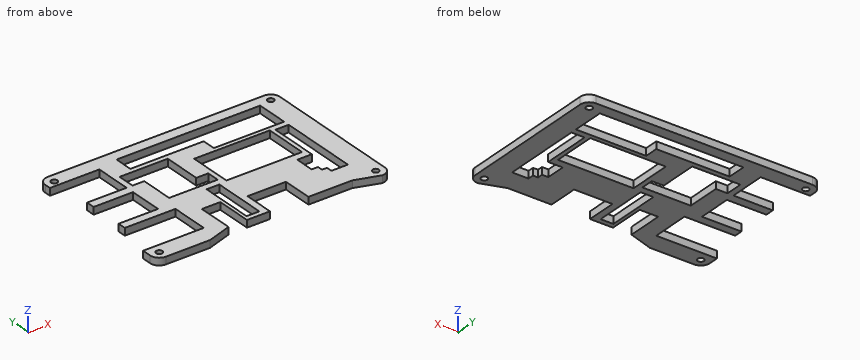
```python
from build123d import *

# Parameters (mm, degrees)
SKETCH2_W           = 5.4034
SKETCH2_H           = 22.6066
SKETCH2_W_2         = 31.9679
SKETCH2_H_2         = 18.2371
BOSS_EXTRUDE1_DEPTH = 3.048
SKETCH3_R           = 1.338245378
CUT_EXTRUDE1_DEPTH  = 72.310891511


with BuildPart() as part:
    # Sketch2 → Boss-Extrude1 (new body)
    with BuildSketch(Plane(origin=(0, 0, 8.171752382), x_dir=(-1, 0, 0), z_dir=(0, 0, -1))):
        with BuildLine():
            Line((-23.844892625, -33.084405696), (-34.084892625, -36.451005696))
            ThreePointArc((-34.084892625, -36.451005696), (-36.778969461, -35.335082532), (-37.894892625, -32.641005696))
            Line((-37.894892625, -32.641005696), (-37.894892625, 26.697694304))
            ThreePointArc((-37.894892625, 26.697694304), (-36.778969461, 29.391771141), (-34.084892625, 30.507694304))
            Line((-34.084892625, 30.507694304), (57.404932375, 30.507694304))
            ThreePointArc((57.404932375, 30.507694304), (60.103884597, 29.386886916), (61.214907375, 26.683892153))
            Line((61.214907375, 26.683892153), (61.214907375, 24.068294304))
            Line((61.214907375, 24.068294304), (40.325007375, 24.068294304))
            Line((40.325007375, 24.068294304), (40.325007375, 8.658194304))
            Line((40.325007375, 8.658194304), (56.975007375, 8.658194304))
            Line((56.975007375, 8.658194304), (56.975007375, 4.997894304))
            Line((56.975007375, 4.997894304), (40.325007375, 4.997894304))
            Line((40.325007375, 4.997894304), (40.325007375, -9.121805696))
            Line((40.325007375, -9.121805696), (56.975007375, -9.121805696))
            Line((56.975007375, -9.121805696), (56.975007375, -12.628005696))
            Line((56.975007375, -12.628005696), (35.575007375, -12.628005696))
            Line((35.575007375, -12.628005696), (35.575007375, -28.627805696))
            Line((35.575007375, -28.627805696), (61.214907375, -28.627805696))
            Line((61.214907375, -28.627805696), (61.214907375, -32.613401529))
            ThreePointArc((61.214907375, -32.613401529), (60.108826144, -35.325305244), (57.405007375, -36.451005696))
            Line((57.405007375, -36.451005696), (38.714307375, -36.451005696))
            Line((38.714307375, -36.451005696), (28.474307375, -33.084405696))
            Line((28.474307375, -33.084405696), (28.474307375, -18.034905696))
            Line((28.474307375, -18.034905696), (20.658107375, -18.034905696))
            Line((20.658107375, -18.034905696), (20.658107375, -33.084405696))
            Line((20.658107375, -33.084405696), (10.926407375, -33.084405696))
            Line((10.926407375, -33.084405696), (10.926407375, -20.384405696))
            Line((10.926407375, -20.384405696), (-5.302892625, -20.384405696))
            Line((-5.302892625, -20.384405696), (-5.302892625, -33.084405696))
            Line((-5.302892625, -33.084405696), (-23.844892625, -33.084405696))
        make_face()
        with Locations((16.546707375, -19.663505696)):
            Rectangle(SKETCH2_W, SKETCH2_H, mode=Mode.SUBTRACT)
        Polygon((-29.004892625, -23.698905696), (-22.066892625, -23.698905696), (-22.066892625, -21.185805696), (-19.950892625, -21.185805696), (-19.950892625, -18.920605696), (-17.244692625, -18.920605696), (-17.244692625, -10.792605696), (-23.416892625, -10.792605696), (-23.416892625, 9.801194304), (-29.004892625, 9.801194304), align=None, mode=Mode.SUBTRACT)
        with Locations((-5.654942625, 1.475544304)):
            Rectangle(SKETCH2_W_2, SKETCH2_H_2, mode=Mode.SUBTRACT)
        Polygon((12.361007375, -0.097605696), (17.441007375, -0.097605696), (17.441007375, 15.972394304), (37.825007375, 15.972394304), (37.825007375, 8.658194304), (32.872007375, 8.658194304), (32.872007375, -5.431505696), (12.361007375, -5.431505696), align=None, mode=Mode.SUBTRACT)
        Polygon((0.677107375, 12.372094304), (-29.004794688, 12.372094304), (-29.004892625, 25.896994304), (31.688307375, 25.896994304), (31.688307375, 18.086994304), (0.677107375, 18.086994304), align=None, mode=Mode.SUBTRACT)
    extrude(amount=BOSS_EXTRUDE1_DEPTH)

    # Sketch3 → Cut-Extrude1 (cut, through all)
    with BuildSketch(Plane(origin=(0, 0, 5.123752382), x_dir=(-1, 0, 0), z_dir=(0, 0, -1))):
        with Locations((57.405007375, -32.641005696)):
            Circle(SKETCH3_R)
        with Locations((-34.084892625, -32.641005696)):
            Circle(SKETCH3_R)
        with Locations((-34.084892625, 26.697694304)):
            Circle(SKETCH3_R)
        with Locations((57.404932375, 26.697694304)):
            Circle(SKETCH3_R)
    extrude(amount=-CUT_EXTRUDE1_DEPTH, mode=Mode.SUBTRACT)


solid = part.part
```
Build history of the part. All positions in model axes, mm. Round coordinates to 2 decimals unless told otherwise and drop trailing zeros. Write each loop counter-clockwise with the first axis right and the second up, starting at its lowest first coordinate (ties: lowest second). Pieces come first, ordered by that corner, then holes.
1) Band-saw the part on A-A, the plane x = 8. List the corners of the cut face in (y, z), and give its area (3 significant figures).
2) Band-saw the part on B-B, the plane y = -22.5. List the corners of the cut face in (x, z) (3 decimals), and give its area (3 significant figures).
3) Band-saw the part on D-D, the plane x = -8. List the corners of the cut face in (y, z), and give its area (3 significant figures).
4) Band-saw the part on C-C, the plane y = 21.5. List the corners of the cut face in (x, z) (3 decimals), and give its area (3 significant figures).
5) Drill centre lines: probe 1 along X at (y, z) = (8.5, 6.55) (3 decimals); probe 2 along X at (y, z) = (-4, 6.45) (3 decimals); probe 3 along Y at (x, z) = (16.5, 7.8). Where is each one in solid material? Low to high.
6) Pin check, flat tips, straight feed: pin 1 (8 mm diameter, centred on x = -18, y = -19.5, fed in from -Z); pin 2 (1.5 mm diameter, centred on x = -15, z = 6, fed in from -Y); pin 3 (1.5 mm diameter, centred on x = -31.5, z = 6, fed in from -Y); pin 4 (0.9 mm diameter, centred on x = -23, z = 7, fed in from -Y). Stop position of each tip, or through.
Ans:
1. outline: (-33.08, 5.12) - (-7.64, 5.12) - (-7.64, 8.17) - (-33.08, 8.17) - close; (10.59, 5.12) - (12.37, 5.12) - (12.37, 8.17) - (10.59, 8.17) - close; (25.9, 5.12) - (30.51, 5.12) - (30.51, 8.17) - (25.9, 8.17) - close
1. area: 97.0 mm2
2. outline: (-35.575, 5.124) - (-28.474, 5.124) - (-28.474, 8.172) - (-35.575, 8.172) - close; (-20.658, 5.124) - (-19.248, 5.124) - (-19.248, 8.172) - (-20.658, 8.172) - close; (-13.845, 5.124) - (-10.926, 5.124) - (-10.926, 8.172) - (-13.845, 8.172) - close; (5.303, 5.124) - (22.067, 5.124) - (22.067, 8.172) - (5.303, 8.172) - close; (29.005, 5.124) - (37.895, 5.124) - (37.895, 8.172) - (29.005, 8.172) - close
2. area: 113 mm2
3. outline: (-20.38, 5.12) - (-7.64, 5.12) - (-7.64, 8.17) - (-20.38, 8.17) - close; (10.59, 5.12) - (18.09, 5.12) - (18.09, 8.17) - (10.59, 8.17) - close; (25.9, 5.12) - (30.51, 5.12) - (30.51, 8.17) - (25.9, 8.17) - close
3. area: 75.7 mm2
4. outline: (-40.325, 5.124) - (-31.688, 5.124) - (-31.688, 8.172) - (-40.325, 8.172) - close; (29.005, 5.124) - (37.895, 5.124) - (37.895, 8.172) - (29.005, 8.172) - close
4. area: 53.4 mm2
5. probe 1: x = -56.975 to -32.872, -17.441 to -10.329, 21.639 to 23.417, 29.005 to 37.895
5. probe 2: x = -40.325 to -32.872, -12.361 to -10.329, 21.639 to 23.417, 29.005 to 37.895
5. probe 3: y = -33.08 to -7.64, 10.59 to 12.37, 25.9 to 30.51
6. pin 1: stops at z = 5.12
6. pin 2: stops at y = -33.08
6. pin 3: stops at y = -34.33
6. pin 4: stops at y = -18.03
